Part model, mm, in its own coordinate system. A direction names the side the tool comes from. Round coordinates to 2 decimals unless told otherwise and drop trailing zeros. One line per question, with ' | ' between items.
from build123d import *

# Parameters (mm, degrees)
BOSS_EXTRUDE1_DEPTH     = 10
CUT_EXTRUDE1_DEPTH      = 229.503191587
CUT_EXTRUDE1_DEPTH_BACK = 229.503191587
SKETCH2_R               = 7.5
CUT_EXTRUDE4_DEPTH      = 2
FILLET3_R               = 6


with BuildPart() as part:
    # Sketch1 → Boss-Extrude1 (new body)
    with BuildSketch(Plane(origin=(0, 0, 0), x_dir=(0, 0, -1), z_dir=(1, 0, 0))):
        with BuildLine():
            ThreePointArc((11.970705016, -32.889241728), (31.720772546, 14.791639161), (-17.5, 30.310889132))
            add(Edge.make_bspline(
                [(-17.5, 30.310889132), (-34.321955695, 20.598728483), (-116.723953626, -40.410250972), (-156.313763477, -126.034194964), (-159.547511978, -132.968991002)],
                knots=[0, 0, 0, 0, 0.889912334, 1, 1, 1, 1], degree=3))
            ThreePointArc((-159.547511978, -132.968991002), (-152.167348404, -158.289185154), (-126.100467375, -154.277108431))
            add(Edge.make_bspline(
                [(-126.100467375, -154.277108431), (-80.64177253, -100.101545535), (-58.2293325, -84.719492888), (-25.919121569, -50.790307967), (-14.885033301, -42.663931094), (11.970705016, -32.889241728)],
                knots=[0, 0, 0, 0, 0.511217005, 0.600270542, 0.89053537, 0.89053537, 0.89053537, 0.89053537], degree=3))
        make_face()
    extrude(amount=BOSS_EXTRUDE1_DEPTH)

    # Sketch2 → Cut-Extrude1 (cut, two sides: drawn at the far end of the back side and taken through both)
    with BuildSketch(Plane(origin=(10, 0, 0), x_dir=(0, 0, -1), z_dir=(1, 0, 0)).offset(-CUT_EXTRUDE1_DEPTH_BACK)):
        Circle(SKETCH2_R)
        with Locations((-141.421356237, -141.421356237)):
            Circle(SKETCH2_R)
    extrude(amount=CUT_EXTRUDE1_DEPTH + CUT_EXTRUDE1_DEPTH_BACK, mode=Mode.SUBTRACT)

    # Sketch8 → Cut-Extrude4 (cut)
    with BuildSketch(Plane(origin=(10, 0, 0), x_dir=(0, 0, -1), z_dir=(1, 0, 0))):
        with BuildLine():
            ThreePointArc((5.301312222, -14.565235622), (-14.047770699, -6.550583057), (-7.75, 13.423393759))
            Line((-7.75, 13.423393759), (-13.270700045, 22.985526729))
            Line((-13.270700045, 22.985526729), (-13.5, 23.382685902))
            add(Edge.make_bspline(
                [(-13.5, 23.382685902), (-14.004264792, 23.091548489), (-14.596989898, 22.736556542), (-15.930761723, 21.910191472), (-16.672259928, 21.43865672), (-19.096143962, 19.858481722), (-20.97746579, 18.58453004), (-23.985838626, 16.468739554), (-24.932203297, 15.79405814), (-25.916949038, 15.082203502)],
                knots=[0, 0, 0, 0, 0.03125, 0.03125, 0.0625, 0.0625, 0.125, 0.125, 0.151902129, 0.151902129, 0.151902129, 0.151902129], degree=3))
            add(Edge.make_bspline(
                [(-25.916949038, 15.082203502), (-29.507797216, 12.4864452), (-33.608989313, 9.396403406), (-49.503275079, -3.177533176), (-63.377476055, -15.156595083), (-91.964800189, -43.803959857), (-106.678912673, -60.475554794), (-126.373284326, -88.065760368), (-132.542324418, -97.692221413), (-138.762340902, -108.912812223), (-139.443275699, -110.164633361), (-140.784992316, -112.680202379), (-141.44751941, -113.947019213), (-143.40368157, -117.749366226), (-144.665797353, -120.286656297), (-146.645761611, -124.353749783), (-147.397332853, -125.92044903), (-148.121316458, -127.444213001)],
                knots=[0.151902129, 0.151902129, 0.151902129, 0.151902129, 0.25, 0.25, 0.5, 0.5, 0.75, 0.75, 0.875, 0.875, 0.890625, 0.890625, 0.90625, 0.90625, 0.9375, 0.9375, 0.957617953, 0.957617953, 0.957617953, 0.957617953], degree=3))
            ThreePointArc((-148.121316458, -127.444213001), (-133.163008443, -128.304584847), (-125.921356237, -141.421356237))
            ThreePointArc((-125.921356237, -141.421356237), (-125.921911553, -141.552560245), (-125.923577462, -141.683754851))
            add(Edge.make_bspline(
                [(-125.923577462, -141.683754851), (-118.529925562, -133.022812133), (-111.861983926, -125.488119901), (-98.042519438, -110.377224048), (-91.266586508, -103.365591459), (-79.155605263, -91.336141526), (-73.820810692, -86.318727269), (-66.552703556, -79.612530547), (-64.252740209, -77.514005309), (-59.839444304, -73.477424972), (-57.726273613, -71.539479143), (-53.620860933, -67.706762992), (-51.628593649, -65.812039684), (-49.166594827, -63.393004096), (-48.676627606, -62.907593959), (-47.692724643, -61.92458048), (-47.198430387, -61.426856534), (-45.710588093, -59.921105575), (-44.712177008, -58.90055567), (-42.710952583, -56.857105325), (-41.708160185, -55.834215393), (-39.703469442, -53.815256413), (-38.703400895, -52.821019854), (-35.691473525, -49.90421685), (-33.653791845, -48.033660498), (-29.262128181, -44.400093328), (-26.909957963, -42.640832773), (-21.694579862, -39.210652351), (-18.834074142, -37.540197568), (-12.384697646, -34.20169183), (-8.795186024, -32.532039364), (-0.610596797, -29.072552339), (3.985554691, -27.282176582), (9.23454387, -25.371700761)],
                knots=[0.027086016, 0.027086016, 0.027086016, 0.027086016, 0.125, 0.125, 0.25, 0.25, 0.375, 0.375, 0.4375, 0.4375, 0.5, 0.5, 0.5625, 0.5625, 0.578125, 0.578125, 0.59375, 0.59375, 0.625, 0.625, 0.65625, 0.65625, 0.6875, 0.6875, 0.75, 0.75, 0.8125, 0.8125, 0.875, 0.875, 0.9375, 0.9375, 1, 1, 1, 1], degree=3))
            Line((9.23454387, -25.371700761), (5.301312222, -14.565235622))
        make_face()
    cut_extrude4 = extrude(amount=-CUT_EXTRUDE4_DEPTH, mode=Mode.SUBTRACT)

    # Fillet3
    fillet3_edges = [part.edges().sort_by_distance(p)[0] for p in [
        (9, -25.371700761, -9.23454387),
        (9, -14.565235622, -5.301312222),
        (9, 13.423393759, 7.75),
        (9, 23.382685902, 13.5),
        (9, -141.683754851, 125.923577462),
        (9, -127.444213001, 148.121316458),
    ]]
    fillet(fillet3_edges, radius=FILLET3_R)

    # Mirror1: Cut-Extrude4 across plane
    add(cut_extrude4.mirror(Plane(origin=(5, 0, 0), x_dir=(0, 0, 1), z_dir=(1, 0, 0))), mode=Mode.SUBTRACT)


solid = part.part
1) Probe line 1 (Y direction, x = 6.25, z = 0); line 2 (Z direction, x = 3.25, y = 0); line 3 (Y direction, x = 7, z = 142). List the from-to ranges inside material, lowest first. Write a range as [from, to].
The answers:
line 1: y = [-37.51, -7.5], [7.5, 35] | line 2: z = [-35, -7.5], [7.5, 57.71] | line 3: y = [-161.41, -148.9], [-133.94, -98.39]
2) Drop flat-ended pins along their axis: pin 1 (1 mm diameter, centred on x = 1.5, z = 134.5, fed in from -Y); pin 2 (1.5 mm diameter, centred on x = 7, z = 56, fed in from -Y); pin 3 (9 mm diameter, centred on y = -141.42, z = 141.42, fed in from -X); pin 4 (5 mm diameter, centred on x = 8, y = -34, fed in from +Z). Give the stop position or say it passes through.
The answers:
pin 1: stops at y = -160.36 | pin 2: stops at y = -81.49 | pin 3: passes through | pin 4: stops at z = 95.5
3) Which spindle directions (+Z, -Z, +X, -X, +Y, -Y) get a long thin tool onto all of the face, cutting with end or side? Do faces 1 (the face through (4.93, -145.985, 147.373)), 2 (the face through (2, -53, 70)), 3 (the face through (8, -51, 69)). Say none if no direction does.
The answers:
face 1: +X, -X | face 2: -X | face 3: +X
4) Saw through at A-A (x = 5.5). Give the number of separate pieces and of enclosed holes in the cut face, plus the area to 3 significant figures.
The answers:
separate pieces: 1 | enclosed holes: 2 | area: 13,700 mm²
5) Two-plate mould, pull along Z, no slides. Class faces 4 (the face through (4.93, -158.069, 152.505)), 5 (the face through (0, -63, 42)), 6 (the face through (0.99, -6.84, 13.91)): released by +Z, released by -Z, zero draft, split by the parting line, or undercut.
The answers:
face 4: split by the parting line | face 5: zero draft | face 6: undercut
